```python
from build123d import *

# Parameters (mm, degrees)
F0_W     = 584.2
F0_H     = 219.71
F1_DEPTH = 5.334
F2_W     = 571.5
F2_H     = 213.36
F2_W_2   = 546.1
F2_H_2   = 187.96
F3_DEPTH = 12.7
F4_R     = 25.4
F6_DEPTH = 12.7
F8_DEPTH = 5.334
F9_DEPTH = 5.334


# Not quite as in the source:
# - a feature names something its author has since deleted; it is built from what else it names


with BuildPart() as f1:
    # F0 (on Front) → F1 (new body)
    with BuildSketch(Plane.XZ):
        with Locations((-292.1, 109.855)):
            Rectangle(F0_W, F0_H)
    extrude(amount=F1_DEPTH)

    # F2 (on face) → F3 (join)
    with BuildSketch(Plane.XZ.offset(5.334)):
        with Locations((-292.1, 113.03)):
            Rectangle(F2_W, F2_H)
        with Locations((-292.1, 113.03)):
            Rectangle(F2_W_2, F2_H_2, mode=Mode.SUBTRACT)
    extrude(amount=F3_DEPTH)

    # F4
    f4_edges = [f1.edges().sort_by_distance(p)[0] for p in [
        (-565.15, -11.684, 207.01),
        (-19.05, -11.684, 207.01),
        (-19.05, -11.684, 19.05),
        (-565.15, -11.684, 19.05),
    ]]
    fillet(f4_edges, radius=F4_R)

    # F5 (on face) → F6 (cut)
    with BuildSketch(Plane.XZ.offset(18.034)):
        Polygon((-118.11, 219.71), (-125.73, 207.01), (-118.11, 207.01), (-113.5820166854, 214.5566388576), (-110.49, 219.71), align=None)
        Polygon((-56.5979833146, 214.5566388576), (-52.07, 207.01), (-44.45, 207.01), (-52.07, 219.71), (-59.69, 219.71), align=None)
        Polygon((-59.69, 219.71), (-110.49, 219.71), (-113.5820166854, 214.5566388576), (-56.5979833146, 214.5566388576), align=None)
    extrude(amount=-F6_DEPTH, mode=Mode.SUBTRACT)

    # F7 (on face) → F8 (cut)
    with BuildSketch(Plane(origin=(0, 0, 0), x_dir=(-1, 0, 0), z_dir=(0, 1, 0))):
        with BuildLine():
            add(Edge.make_bspline(
                [(292.1, 6.35), (289.8878914708, 4.2388101088), (287.6757829415, 2.1276202176), (285.3383261504, 0)],
                knots=[0, 0, 0, 0, 0.0566650496, 0.0566650496, 0.0566650496, 0.0566650496], degree=3))
            Line((285.3383261504, 0), (292.1, 0))
            Line((292.1, 0), (292.1, 6.35))
        make_face()
        with BuildLine():
            add(Edge.make_bspline(
                [(292.1, 6.35), (294.3115112442, 4.2388053382), (296.5230224884, 2.1276106765), (298.8599853109, 0)],
                knots=[0, 0, 0, 0, 0.056662645, 0.056662645, 0.056662645, 0.056662645], degree=3))
            Line((292.1, 6.35), (292.1, 0))
            Line((292.1, 0), (298.8599853109, 0))
        make_face()
    extrude(amount=-F8_DEPTH, mode=Mode.SUBTRACT)

    # F7 (on face) → F9 (join)
    with BuildSketch(Plane(origin=(0, 0, 0), x_dir=(-1, 0, 0), z_dir=(0, 1, 0))):
        with BuildLine():
            Line((285.3383261504, 0), (0, 0))
            add(Edge.make_bspline(
                [(35.5548654074, -18.4164866805), (23.6750755263, -12.5314961521), (11.8375377632, -6.265748076), (0, 0)],
                knots=[0.8952858021, 0.8952858021, 0.8952858021, 0.8952858021, 1, 1, 1, 1], degree=3))
            Line((35.5548654074, -18.4164866805), (260.35, -18.4164866805))
            add(Edge.make_bspline(
                [(285.3383261504, 0), (278.8607301271, -5.8960937002), (271.4205053001, -11.9183662972), (260.35, -18.4164866805)],
                knots=[0.0566650496, 0.0566650496, 0.0566650496, 0.0566650496, 0.2136961022, 0.2136961022, 0.2136961022, 0.2136961022], degree=3))
        make_face()
        with BuildLine():
            add(Edge.make_bspline(
                [(0, 0), (-2.5016001756, 37.5778391816), (-5.0032003512, 75.1556783631), (-5.08, 111.5191693883)],
                knots=[0, 0, 0, 0, 0.4959951232, 0.4959951232, 0.4959951232, 0.4959951232], degree=3))
            Line((0, 0), (0, 219.71))
            add(Edge.make_bspline(
                [(-5.08, 114.935), (-5.0035853497, 150.6697582461), (-2.5017926748, 185.189879123), (0, 219.71)],
                knots=[0.5115421197, 0.5115421197, 0.5115421197, 0.5115421197, 1, 1, 1, 1], degree=3))
            Line((-5.08, 114.935), (-5.08, 111.5191693883))
        make_face()
        with BuildLine():
            Line((260.35, -18.4164866805), (35.5548654074, -18.4164866805))
            add(Edge.make_bspline(
                [(143.5928555626, -50.8), (106.470496214, -50.0055886792), (70.8264502644, -35.8892656507), (35.5548654074, -18.4164866805)],
                knots=[0.5843850409, 0.5843850409, 0.5843850409, 0.5843850409, 0.8952858021, 0.8952858021, 0.8952858021, 0.8952858021], degree=3))
            Line((143.5928555626, -50.8), (150.3785817486, -50.8))
            add(Edge.make_bspline(
                [(260.35, -18.4164866805), (235.5497171967, -32.973656279), (192.5306851802, -49.9188924594), (150.3785817486, -50.8)],
                knots=[0.2136961022, 0.2136961022, 0.2136961022, 0.2136961022, 0.5654790071, 0.5654790071, 0.5654790071, 0.5654790071], degree=3))
        make_face()
        with BuildLine():
            add(Edge.make_bspline(
                [(11.7731056729, 229.2938254471), (8.1151931686, 226.4637173569), (4.2088787391, 223.2851496368), (0, 219.71)],
                knots=[0.9578423111, 0.9578423111, 0.9578423111, 0.9578423111, 1, 1, 1, 1], degree=3))
            Line((0, 219.71), (292.1, 219.71))
            Line((292.1, 219.71), (11.7731056729, 229.2938254471))
        make_face()
        with BuildLine():
            add(Edge.make_bspline(
                [(12.5206463088, 229.87), (12.2726179558, 229.6795636028), (12.0234435309, 229.4875105602), (11.7731056729, 229.2938254471)],
                knots=[0.9549571504, 0.9549571504, 0.9549571504, 0.9549571504, 0.9578423111, 0.9578423111, 0.9578423111, 0.9578423111], degree=3))
            Line((11.7731056729, 229.2938254471), (292.1, 219.71))
            Line((292.1, 219.71), (573.1817260974, 229.3196316614))
            add(Edge.make_bspline(
                [(572.5320605941, 229.87), (572.7473841939, 229.6879525114), (572.9639346328, 229.5045002197), (573.1817260974, 229.3196316614)],
                knots=[0.9616983958, 0.9616983958, 0.9616983958, 0.9616983958, 0.9640299265, 0.9640299265, 0.9640299265, 0.9640299265], degree=3))
            Line((572.5320605941, 229.87), (514.35, 229.87))
            Line((514.35, 229.87), (292.1, 229.87))
            Line((292.1, 229.87), (82.55, 229.87))
            Line((82.55, 229.87), (12.5206463088, 229.87))
        make_face()
        with BuildLine():
            Line((573.1817260974, 229.3196316614), (292.1, 219.71))
            Line((292.1, 219.71), (584.2, 219.71))
            add(Edge.make_bspline(
                [(573.1817260974, 229.3196316614), (576.5417396252, 226.4675416698), (580.1971331881, 223.2783621084), (584.2, 219.71)],
                knots=[0.9640299265, 0.9640299265, 0.9640299265, 0.9640299265, 1, 1, 1, 1], degree=3))
        make_face()
        with BuildLine():
            add(Edge.make_bspline(
                [(298.8599853109, 0), (305.3364495341, -5.8962831133), (312.7764065366, -11.9186444461), (323.85, -18.4164866805)],
                knots=[0.056662645, 0.056662645, 0.056662645, 0.056662645, 0.2136927825, 0.2136927825, 0.2136927825, 0.2136927825], degree=3))
            Line((323.85, -18.4164866805), (548.6673215949, -18.4164866805))
            add(Edge.make_bspline(
                [(548.6673215949, -18.4164866805), (560.540064076, -12.5314899408), (572.370032038, -6.2657449704), (584.2, 0)],
                knots=[0.8952964295, 0.8952964295, 0.8952964295, 0.8952964295, 1, 1, 1, 1], degree=3))
            Line((584.2, 0), (298.8599853109, 0))
        make_face()
        with BuildLine():
            Line((548.6673215949, -18.4164866805), (323.85, -18.4164866805))
            add(Edge.make_bspline(
                [(323.85, -18.4164866805), (348.6543054028, -32.9713340996), (391.6899454814, -49.9118498543), (433.8458201185, -50.8)],
                knots=[0.2136927825, 0.2136927825, 0.2136927825, 0.2136927825, 0.5654325768, 0.5654325768, 0.5654325768, 0.5654325768], degree=3))
            Line((433.8458201185, -50.8), (440.69, -50.8))
            add(Edge.make_bspline(
                [(440.69, -50.8), (477.8051745876, -49.9992725657), (513.4246952416, -35.8853016167), (548.6673215949, -18.4164866805)],
                knots=[0.5844980763, 0.5844980763, 0.5844980763, 0.5844980763, 0.8952964295, 0.8952964295, 0.8952964295, 0.8952964295], degree=3))
        make_face()
        with BuildLine():
            add(Edge.make_bspline(
                [(82.55, 255.27), (55.6261452853, 252.2921647864), (42.3764019315, 252.7932765823), (12.5206463088, 229.87)],
                knots=[0.6076635734, 0.6076635734, 0.6076635734, 0.6076635734, 0.9549571504, 0.9549571504, 0.9549571504, 0.9549571504], degree=3))
            Line((12.5206463088, 229.87), (82.55, 229.87))
            Line((82.55, 229.87), (82.55, 255.27))
        make_face()
        with BuildLine():
            add(Edge.make_bspline(
                [(589.28, 114.935), (589.2035853497, 150.6697582461), (586.7017926748, 185.189879123), (584.2, 219.71)],
                knots=[0.5115421197, 0.5115421197, 0.5115421197, 0.5115421197, 1, 1, 1, 1], degree=3))
            Line((584.2, 219.71), (584.2, 0))
            add(Edge.make_bspline(
                [(584.2, 0), (586.7016001756, 37.5778391816), (589.2032003512, 75.1556783632), (589.28, 111.5191693884)],
                knots=[0, 0, 0, 0, 0.4959951232, 0.4959951232, 0.4959951232, 0.4959951232], degree=3))
            Line((589.28, 111.5191693884), (589.28, 114.935))
        make_face()
        with BuildLine():
            Line((82.55, 255.27), (82.55, 229.87))
            Line((82.55, 229.87), (292.1, 229.87))
            Line((292.1, 229.87), (292.1, 306.07))
            add(Edge.make_bspline(
                [(292.1, 306.07), (218.631118536, 276.3414680958), (129.6589788413, 260.4803525873), (82.55, 255.27)],
                knots=[0, 0, 0, 0, 0.6076635734, 0.6076635734, 0.6076635734, 0.6076635734], degree=3))
        make_face()
        with BuildLine():
            Line((514.35, 229.87), (572.5320605941, 229.87))
            add(Edge.make_bspline(
                [(514.35, 255.27), (536.1096268059, 253.2414037435), (541.9337770664, 255.7396244938), (572.5320605941, 229.87)],
                knots=[0.6303792087, 0.6303792087, 0.6303792087, 0.6303792087, 0.9616983958, 0.9616983958, 0.9616983958, 0.9616983958], degree=3))
            Line((514.35, 255.27), (514.35, 229.87))
        make_face()
        with BuildLine():
            Line((292.1, 306.07), (292.1, 229.87))
            Line((292.1, 229.87), (514.35, 229.87))
            Line((514.35, 229.87), (514.35, 255.27))
            add(Edge.make_bspline(
                [(292.1, 306.07), (373.8620877266, 279.3765068054), (472.9493903602, 259.129676569), (514.35, 255.27)],
                knots=[0, 0, 0, 0, 0.6303792087, 0.6303792087, 0.6303792087, 0.6303792087], degree=3))
        make_face()
    extrude(amount=-F9_DEPTH)


solid = f1.part
```
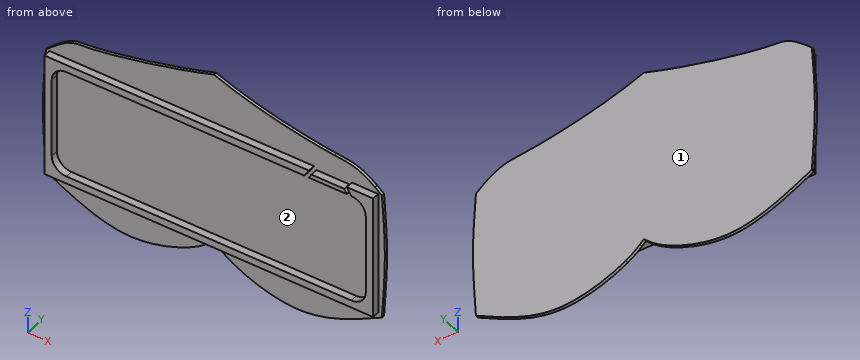
The listing builds one solid part. Answer for the finished solid, in the listing's coordinates (mm). Face numbers are marked on the shaded views. Give positions to 0.01 mm unless a question says otherwise; leave off trailing zeros. Loops run counter-clockwise (first coordinate to the right, second up) from the corner with the lowest first, then second, coordinate; pieces in that order, holes last. Notation, with made-up numbers: M 42.25,65.25 L 80.25,65.25 A28 cw 80.25,83.25 Z; hole C -33,-24 d9. An arc over 180 degrees is marked long. One line per item, written item: value.
1. Section A-A on y = -8.5 is taken. Determine the outline of the cut face in (x, z), plus the area to 3 significant figures.
Found:
outline: M -577.85,6.35 L -6.35,6.35 L -6.35,219.71 L -52.07,219.71 L -44.45,207.01 A25.4 cw -19.05,181.61 L -19.05,44.45 A25.4 cw -44.45,19.05 L -539.75,19.05 A25.4 cw -565.15,44.45 L -565.15,181.61 A25.4 cw -539.75,207.01 L -125.73,207.01 L -118.11,219.71 L -577.85,219.71 Z; M -118.11,207.01 L -52.07,207.01 L -56.6,214.56 L -113.58,214.56 Z
area: 19,400 mm^2
2. Find the intervals of material crossed by probe 1 along Z at (x, y) = (-75, -13.5); probe 2 along Z at (x, y) = (-299, -12.25); probe 3 along X at (y, z) = (-15.25, 47), in increasing order.
Found:
probe 1: 6.35 to 19.05, 207.01 to 214.56
probe 2: 6.35 to 19.05, 207.01 to 219.71
probe 3: -577.85 to -565.15, -19.05 to -6.35
3. For a pull along X with two mould halves and no side action, classify the marked faces 1 and 2 as pulls with the +X half, pulls with the -X half, needs draft (parallel to the pull), parting line crosses it, or undercut.
Found:
face 1: needs draft
face 2: undercut
4. Each of these flat-tipped pins is pushed along its axis until it touches: P1, Ø2, axis at x = -277.5, z = 4, coming from the -Y side; P2, Ø6.5, axis at y = -12, z = 100, coming from the +X side; P3, Ø2, axis at x = -247, y = -14.5, coming from the -Z side; P4, Ø10, axis at x = -344, z = 99.5, coming from the +Y side. Where does it stop, or does it pass through?
Found:
P1: y = -5.33
P2: x = -6.35
P3: z = 6.35
P4: y = 0
